from build123d import *

# Parameters (mm, degrees)
SKETCH3_R                 = 4.7625
OXIDIZER_INLET_HOLE_DEPTH = 37.83
FLANGE_HOLES_D            = 5.1054
FLANGE_HOLES_DEPTH        = 22.225
DOWEL_HOLES_D             = 4.7625
DOWEL_HOLES_DEPTH         = 6.35
DOWEL_HOLES_TIP           = 1.430799349
SKETCH12_R                = 28.575
CUT_EXTRUDE2_DEPTH        = 9.525
SKETCH16_R                = 28.575
SKETCH17_R                = 4.7625
CIRPATTERN1_COUNT         = 8
FILLET1_R                 = 1.27


with BuildPart() as part:
    # Sketch2 → Main Structure (revolve)
    with BuildSketch(Plane.XY):
        Polygon((41.355, 13.081), (41.355, 6.2484), (46.355, 6.2484), (46.355, 0), (9.525, 0), (9.525, 63.5), (31.75, 63.5), (31.75, 13.081), align=None)
    revolve(axis=Axis((9.525, 0, 0), (1, 0, 0)))

    # Sketch3 → Oxidizer Inlet Hole (cut, through all)
    with BuildSketch(Plane(origin=(46.355, 0, 0), x_dir=(0, 0, -1), z_dir=(1, 0, 0))):
        Circle(SKETCH3_R)
    extrude(amount=-OXIDIZER_INLET_HOLE_DEPTH, mode=Mode.SUBTRACT)

    # Flange Holes
    with Locations(Plane(origin=(31.75, 0, 0), x_dir=(0, 0, 1), z_dir=(1, 0, 0))):
        with Locations((0, 58.42), (-29.21, 50.593204089), (-50.593204089, 29.21), (-58.42, 0), (-50.593204089, -29.21), (-29.21, -50.593204089), (0, -58.42), (29.21, -50.593204089), (50.593204089, -29.21), (58.42, 0), (50.593204089, 29.21), (29.21, 50.593204089)):
            Hole(FLANGE_HOLES_D / 2, depth=FLANGE_HOLES_DEPTH)

    # Dowel Holes
    with Locations(Plane.ZY.offset(-9.525)):
        with Locations((56.429386772, -15.120208615), (-56.429386772, 15.120208615)):
            Hole(DOWEL_HOLES_D / 2, depth=DOWEL_HOLES_DEPTH)
            with Locations((0, 0, -(DOWEL_HOLES_DEPTH + DOWEL_HOLES_TIP / 2))):  # 118° drill point
                Cone(0, DOWEL_HOLES_D / 2, DOWEL_HOLES_TIP, mode=Mode.SUBTRACT)

    # Sketch12 → Cut-Extrude2 (cut)
    with BuildSketch(Plane.ZY.offset(-9.525)):
        Circle(SKETCH12_R)
    extrude(amount=-CUT_EXTRUDE2_DEPTH, mode=Mode.SUBTRACT)

    # Sketch16 → Internal Flow Path Loft Cut section 0
    with BuildSketch(Plane.ZY.offset(-19.05)):
        Circle(SKETCH16_R)
    # Sketch17 → Internal Flow Path Loft Cut section 1
    with BuildSketch(Plane.ZY.offset(-30.48)):
        Circle(SKETCH17_R)
    loft(mode=Mode.SUBTRACT)

    # Sketch20 → #4-40 Tapped Hole1 (revolve, cut)
    with BuildSketch(Plane(origin=(9.525, 0, 33.3375), x_dir=(0, 0, 1), z_dir=(0, 1, 0))):
        Polygon((0, 0), (0, 13.887152758), (1.1303, 13.208), (1.1303, 0), align=None)
    f_4_40_tapped_hole1 = revolve(axis=Axis((3.175, 0, 33.3375), (1, 0, 0)), mode=Mode.SUBTRACT)

    # CirPattern1: #4-40 Tapped Hole1 ×8 about axis
    cirpattern1_axis = Axis((0, 0, 0), (1, 0, 0))
    for i in range(1, CIRPATTERN1_COUNT):
        add(f_4_40_tapped_hole1.rotate(cirpattern1_axis, i * 360 / CIRPATTERN1_COUNT), mode=Mode.SUBTRACT)

    # Fillet1
    fillet1_edges = [part.edges().sort_by_distance(p)[0] for p in [
        (31.75, -13.081, 0),
    ]]
    fillet(fillet1_edges, radius=FILLET1_R)


solid = part.part
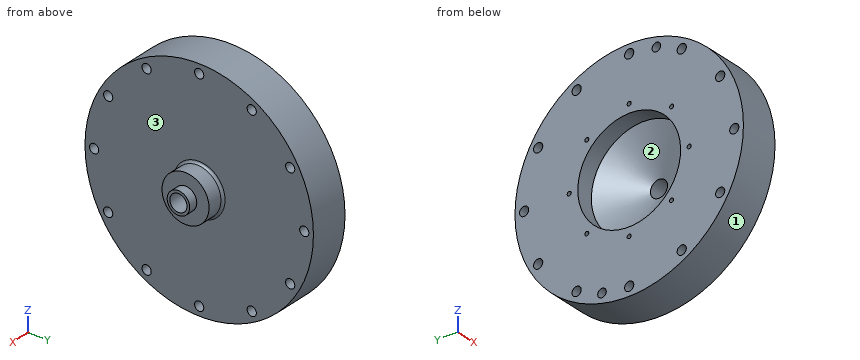
The model under review builds one solid part; all positions refer to its coordinate system, in mm. Face numbers are marked on the shaded views. Round coordinates to 2 decimals unless told otherwise and drop trailing zeros. Loops run counter-clockwise (first coordinate to the right, second up) from the corner with the lowest first, then second, coordinate; pieces in that order, holes last. Notation, with made-up numbers: (36.25, 7) -> (83.25, 7) arc R33 cw to (83.25, 36) -> close; hole circle Ø5 at (-37, 42.25). An arc over 180 degrees is marked (long way). Answer as CSV lines item,"result".
1) Add section A-A on y = 58.42. Write out the cut boundary in (x, z) (3 decimals).
Geometry results:
outline,"(9.525, -24.887) -> (31.75, -24.887) -> (31.75, -2.553) -> (9.525, -2.553) -> close; (9.525, 2.553) -> (31.75, 2.553) -> (31.75, 24.887) -> (9.525, 24.887) -> close"
2) Draft analysis for pull direction Z (two halves, no side actions). For the marked faces 1, 2 and 3, state which applies: pulls with the +Z half, pulls with the -Z half, needs draft (parallel to the pull), parting line crosses it, or undercut.
Geometry results:
face 1,"parting line crosses it"
face 2,"undercut"
face 3,"needs draft"
3) Add section B-B on z = 45. Write out the cut boundary in (x, y) (3 decimals), plus the area to 3 significant figures.
Geometry results:
outline,"(9.525, -44.802) -> (31.75, -44.802) -> (31.75, 44.802) -> (9.525, 44.802) -> close"
area,"1,990 mm²"
4) To check wall thickness, follow line 1 along X through (y, z) = (39, 1) (3 decimals); line 2 along Y through (x, z) = (20.25, -29.21); line 3 along Y through (x, z) = (24.5, -1). State the ranges of each line that lie inside material, in increasing order. Write a range as from..to.
Geometry results:
line 1,"x = 9.525..31.75"
line 2,"y = -56.38..-53.15, -48.04..48.04, 53.15..56.38"
line 3,"y = -63.49..-60.77, -56.07..-17.19, 17.19..56.07, 60.77..63.49"
5) Add section C-C on y = -41. Write out the cut boundary in (x, z) (3 decimals).
Geometry results:
outline,"(9.525, -48.49) -> (31.75, -48.49) -> (31.75, 48.49) -> (9.525, 48.49) -> close"
6) For P1, Ø2, axis at y = 33.34, z = 0, coming from the -X side; P2, Ø1.8, axis at y = 23.57, z = 23.57, coming from the -X side; P3, Ø6, axis at x = 26, z = 46, coming from the +Y side; P4, Ø6.5, axis at y = 50.59, z = -29.21, coming from the -X side (3 decimals), all flat-tipped, find the tip position at first contact; note any pin that passes through.
Geometry results:
P1,"stops at x = 22.81"
P2,"stops at x = 22.87"
P3,"stops at y = 46.73"
P4,"stops at x = 9.525"
